Autodesk Inventor part; units mm, degrees
ref_plane "YZ Plane" through (0, 0, 0) normal (1, 0, 0) x (0, 1, 0)
ref_plane "XZ Plane" through (0, 0, 0) normal (0, 1, 0) x (-1, 0, 0)
ref_plane "XY Plane" through (0, 0, 0) normal (0, 0, 1) x (1, 0, 0)
sketch "Sketch1" plane through (0, 0, 0) normal (0, 1, 0) x (-1, 0, 0)
  circle A0 centre (0, 0) radius 53.975
  circle A1 centre (0, 0) radius 60.325
  dimension "d0" = 107.95
  dimension "d1" = 120.65
extrude "Extrusion1" add sketch "Sketch1" along normal blind 44.45
sketch "Sketch2" plane through (0, 44.45, 0) normal (0, 1, 0) x (1, 0, 0)
  circle A0 centre (0, 0) radius 66.675
  dimension "d4" = 133.35
extrude "Extrusion2" add sketch "Sketch2" along normal blind 44.45
sketch "Sketch3" plane through (0, 44.45, 0) normal (0, -1, 0) x (1, 0, 0)
  circle A0 centre (0, 0) radius 53.975
  dimension "d7" = 107.95
extrude "Extrusion3" cut sketch "Sketch3" against normal blind 31.75
sketch "Sketch4" plane through (0, 88.9, 0) normal (0, 1, 0) x (1, 0, 0)
  circle A0 centre (0, 0) radius 57.15
  dimension "d10" = 114.3
extrude "Extrusion4" add sketch "Sketch4" along normal blind 3.175
sketch "Sketch5" plane through (0, 92.075, 0) normal (0, 1, 0) x (1, 0, 0)
  line L0 (-25.4, -25.4) -> (25.4, -25.4)
  line L1 (25.4, -25.4) -> (25.4, 25.4)
  line L2 (25.4, 25.4) -> (-25.4, 25.4)
  line L3 (-25.4, 25.4) -> (-25.4, -25.4)
  point P0 (0, 0)
  dimension "d13" = 50.8
  dimension "d14" = 50.8
extrude "Extrusion5" add sketch "Sketch5" along normal blind 25.4
fillet "Fillet1" radius 3.175 1 edges at (-66.675, 88.9, 0)
fillet "Fillet2" radius 1.27 1 edges at (-57.15, 92.075, 0)
properties part number "4in Cleanout Adapter w Plug"
For this review, take the finished solid that the model builds, in its own axes (mm). A direction names the side the tool comes from. Round coordinates to 2 decimals unless told otherwise and drop trailing zeros. Write each loop counter-clockwise with the first axis right and the second up, starting at its lowest first coordinate (ties: lowest second). Pieces come first, ordered by that corner, then holes. Notation, with made-up numbers: (20.5, -6.75) - (35.5, -6.75) arc R12 cw to (35.5, 9.25) - close; hole circle Ø3 at (73.25, 83.5). An arc over 180 degrees is marked (long way). Answer as a JSON object with one key per item and string values.
1. For pin 1 Ø10 at (y, z) = (35, -30.5) entering from -X; pin 2 Ø2 at (x, z) = (45, -20.5) entering from -Y; pin 3 Ø3 at (y, z) = (103.5, 19) entering from +X, all flat-tipped, find the tip position at first contact; note any pin that passes through.
Response values:
{"pin 1": "stops at x = -54.67", "pin 2": "stops at y = 76.2", "pin 3": "stops at x = 25.4"}
2. Tool access review of faces 1 (the face through (0, 105, -25.4)), 2 (the face through (-57.095, 89.839, 2.513)), 3 (the face through (0, 105, 25.4)), 4 (the face through (-25.4, 105, 0)), 5 (the face through (60.267, 21.914, -2.652)): name each direction out of +Z, -Z, +X, -X, +Y, -Y from which nothing blocks a thin tool from reaching the whole face with its end or side.
Response values:
{"face 1": "-Z, +X, -X, +Y", "face 2": "+Y", "face 3": "+Z, +X, -X, +Y", "face 4": "+Z, -Z, -X, +Y", "face 5": "-Y"}
3. To check wall thickness, follow line 1 along Z through (x, y) = (0, 69) (3 decimals); line 2 along Z through (x, y) = (0, 20) (3 decimals). State the ranges of each line that lie inside material, in increasing order.
Response values:
{"line 1": "z = -66.675 to -53.975, 53.975 to 66.675", "line 2": "z = -60.325 to -53.975, 53.975 to 60.325"}
4. We need section C-C on y = 64. Give the boundary of the cut face in (x, z) (3 decimals).
Response values:
{"outline": "circle Ø133.35 at (0, 0); hole circle Ø107.95 at (0, 0)"}
5. We need section D-D on y = 81. Give the boundary of the cut face in (x, z) (3 decimals), then the cut area to 3 significant figures.
Response values:
{"outline": "circle Ø133.35 at (0, 0)", "area": "14,000 mm2"}
6. We need section A-A on x = 0. Give the boundary of the cut face in (y, z) (3 decimals), then the cut area to 3 significant figures.
Response values:
{"outline": "(0, -60.325) - (44.45, -60.325) - (44.45, -66.675) - (85.725, -66.675) arc R3.175 ccw to (88.9, -63.5) - (88.9, -57.15) - (90.805, -57.15) arc R1.27 ccw to (92.075, -55.88) - (92.075, -25.4) - (117.475, -25.4) - (117.475, 25.4) - (92.075, 25.4) - (92.075, 55.88) arc R1.27 ccw to (90.805, 57.15) - (88.9, 57.15) - (88.9, 63.5) arc R3.175 ccw to (85.725, 66.675) - (44.45, 66.675) - (44.45, 60.325) - (0, 60.325) - (0, 53.975) - (76.2, 53.975) - (76.2, -53.975) - (0, -53.975) - close", "area": "4,710 mm2"}
7. Draft analysis for pull direction X (two halves, no side actions). For faces 6 (the face through (-1, 76.2, 1)), 7 (the face through (25.4, 105, 0)), 8 (the face through (-57, 88.9, -10)), state which applies: +X half, -X half, draft (parallel to the pull), parting line (faces both ways), or undercut.
Response values:
{"face 6": "undercut", "face 7": "+X half", "face 8": "draft"}
8. We need section B-B on z = 0. Give the boundary of the cut face in (x, y) (3 decimals).
Response values:
{"outline": "(-66.675, 44.45) - (-60.325, 44.45) - (-60.325, 0) - (-53.975, 0) - (-53.975, 76.2) - (53.975, 76.2) - (53.975, 0) - (60.325, 0) - (60.325, 44.45) - (66.675, 44.45) - (66.675, 85.725) arc R3.175 ccw to (63.5, 88.9) - (57.15, 88.9) - (57.15, 90.805) arc R1.27 ccw to (55.88, 92.075) - (25.4, 92.075) - (25.4, 117.475) - (-25.4, 117.475) - (-25.4, 92.075) - (-55.88, 92.075) arc R1.27 ccw to (-57.15, 90.805) - (-57.15, 88.9) - (-63.5, 88.9) arc R3.175 ccw to (-66.675, 85.725) - close"}
